Can you work these out from the model? Positions are in its coordinate system, mm. Face numbers are marked on the shaded views. Round coordinates to 2 decimals unless told otherwise and drop trailing zeros. Order: outer loops, then holes, each group sorted by start corner. A loop starts at its lowest first (then second) coordinate and runs counter-clockwise, first axis right, second up. Notation, with made-up numbers: (87, -28) - (141, -28) arc R15 ccw to (141, -19) - close; hole circle Ø4 at (-20, 37.25). An arc over 180 degrees is marked (long way). Write item = value, one per line.
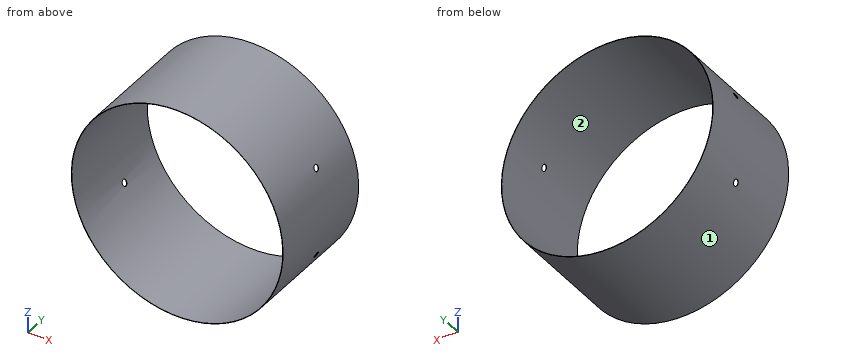
from build123d import *

# Parameters (mm, degrees)
SKETCH1_R               = 501.5
SKETCH1_R_2             = 500
BOSS_EXTRUDE1_DEPTH     = 550
CUT_EXTRUDE2_DEPTH      = 898.499025069
CUT_EXTRUDE2_DEPTH_BACK = 898.499025069
SKETCH2_R               = 13.75


with BuildPart() as part:
    # Sketch1 → Boss-Extrude1 (new body)
    with BuildSketch(Plane(origin=(0, 0, 0), x_dir=(1, 0, 0), z_dir=(0, 1, 0))):
        with Locations(Location((0, 0, 0), (0, 0, 270))):
            Circle(SKETCH1_R)
        with Locations(Location((0, 0, 0), (0, 0, 270))):
            Circle(SKETCH1_R_2, mode=Mode.SUBTRACT)
    extrude(amount=BOSS_EXTRUDE1_DEPTH)

    # Sketch2 → Cut-Extrude2 (cut, two sides: drawn at the far end of the back side and taken through both)
    with BuildSketch(Plane(origin=(0, 0, 0), x_dir=(0, 0, -1), z_dir=(1, 0, 0)).offset(-CUT_EXTRUDE2_DEPTH_BACK)):
        with Locations((211, 312.5)):
            Circle(SKETCH2_R)
        with Locations((-211, 312.5)):
            Circle(SKETCH2_R)
    extrude(amount=CUT_EXTRUDE2_DEPTH + CUT_EXTRUDE2_DEPTH_BACK, mode=Mode.SUBTRACT)


solid = part.part
(1) If we section it at A-A (z = -97): Write out the boundary of the cut face in (x, y).
Computed:
outline = (-492.03, 0) - (-490.5, 0) - (-490.5, 550) - (-492.03, 550) - close; (490.5, 0) - (492.03, 0) - (492.03, 550) - (490.5, 550) - close
(2) If we section it at B-B (x = 25.5): Write out the boundary of the cut face in (y, z).
Computed:
outline = (0, -500.85) - (550, -500.85) - (550, -499.35) - (0, -499.35) - close; (0, 499.35) - (550, 499.35) - (550, 500.85) - (0, 500.85) - close
(3) Thinking about a two-plate mould opening in Z: for the marked faces 1 and 2, which applies, +Z half, -Z half, draft (parallel to the pull), parting line (faces both ways), or undercut?
Computed:
face_1 = parting line
face_2 = undercut
(4) If we section it at C-C (y = 477): Write out the boundary of the cut face in (x, z), plus the area to 3 significant figures.
Computed:
outline = circle Ø1003 at (0, 0); hole circle Ø1000 at (0, 0)
area = 4,720 mm^2
(5) Will these pins go through, and if not, where does the flat tip stop? P1, Ø10, axis at x = -260, y = 212.5, coming from the +Z side; P2, Ø8, axis at y = 304, z = -396.5, coming from the -X side; P3, Ø3, axis at x = -92.5, y = 424, coming from the +Z side.
Computed:
P1 = 431.83
P2 = -312.16
P3 = 493.17
(6) If I drill on line 1 (X direction, y = 416.5, z = 0); line 2 (Z direction, x = 3, y = 218.5); line 3 (X direction, y = 356, z = 15), over which ranges is the centre line in solid material (lowest first)? Write a range as from..to.
Computed:
line_1 = -501.5..-500, 500..501.5
line_2 = -501.49..-499.99, 499.99..501.49
line_3 = -501.28..-499.77, 499.77..501.28
(7) If we section it at D-D (y = 312.5): Write out the boundary of the cut face in (x, z).
Computed:
outline = (-461.08, -197.25) - (-459.45, -197.25) arc R500 cw to (-459.45, 197.25) - (-461.08, 197.25) arc R501.5 ccw to start; (-448.32, -224.75) arc R501.5 ccw to (448.32, -224.75) - (446.64, -224.75) arc R500 cw to (-446.64, -224.75) - close; (-448.32, 224.75) - (-446.64, 224.75) arc R500 cw to (446.64, 224.75) - (448.32, 224.75) arc R501.5 ccw to start; (459.45, -197.25) - (461.08, -197.25) arc R501.5 ccw to (461.08, 197.25) - (459.45, 197.25) arc R500 cw to start
